```python
from build123d import *

# Parameters (mm, degrees)
CROQUIS2_R              = 1.5
SALIENTE_EXTRUIR1_DEPTH = 4
CROQUIS3_R              = 2.85
CORTAR_EXTRUIR1_DEPTH   = 1.65


with BuildPart() as part:
    # Croquis2 → Saliente-Extruir1 (new body)
    with BuildSketch(Plane.XY):
        Polygon((38.497217209, -204.70543153), (46.497217209, -204.70543153), (46.497217209, -193.70543153), (61.497217209, -193.70543153), (61.497217209, -185.70543153), (46.497217209, -185.70543153), (46.497217209, -174.70543153), (38.497217209, -174.70543153), align=None)
        with Locations((42.497217209, -189.70543153)):
            Circle(CROQUIS2_R, mode=Mode.SUBTRACT)
        with Locations((42.497217209, -199.20543153)):
            Circle(CROQUIS2_R, mode=Mode.SUBTRACT)
        with Locations((57.497217209, -189.70543153)):
            Circle(CROQUIS2_R, mode=Mode.SUBTRACT)
        with Locations((49.997217209, -189.70543153)):
            Circle(CROQUIS2_R, mode=Mode.SUBTRACT)
        with Locations((42.497217209, -180.20543153)):
            Circle(CROQUIS2_R, mode=Mode.SUBTRACT)
    extrude(amount=SALIENTE_EXTRUIR1_DEPTH)

    # Croquis3 → Cortar-Extruir1 (cut)
    with BuildSketch(Plane.XY.offset(4)):
        with Locations((42.497217209, -199.20543153)):
            Circle(CROQUIS3_R)
        with Locations((42.497217209, -189.70543153)):
            Circle(CROQUIS3_R)
        with Locations((42.497217209, -180.20543153)):
            Circle(CROQUIS3_R)
        with Locations((49.997217209, -189.70543153)):
            Circle(CROQUIS3_R)
        with Locations((57.497217209, -189.70543153)):
            Circle(CROQUIS3_R)
    extrude(amount=-CORTAR_EXTRUIR1_DEPTH, mode=Mode.SUBTRACT)


solid = part.part
```
The listing builds one solid part. Answer for the finished solid, in the listing's coordinates (mm). A direction names the side the tool comes from. Coordinates: 2 decimals unless noted, no trailing zeros. Loops run counter-clockwise (first coordinate to the right, second up) from the corner with the lowest first, then second, coordinate; pieces in that order, holes last. Notation, with made-up numbers: (-39.75, -38.75) - (-29.75, -38.75) arc R20 ccw to (-29.75, -34.75) - close; hole circle Ø3 at (-13, 46). An arc over 180 degrees is marked (long way). Write item = value, one per line.
1) Section B-B (y = -200) is taken. Determine the outline of the cut face in (x, z), plus the area to 3 significant figures.
Responses:
outline = (38.5, 0) - (41.22, 0) - (41.22, 2.35) - (39.76, 2.35) - (39.76, 4) - (38.5, 4) - close; (43.77, 0) - (46.5, 0) - (46.5, 4) - (45.23, 4) - (45.23, 2.35) - (43.77, 2.35) - close
area = 17.0 mm^2
2) Section D-D (y = -189) is taken. Determine the outline of the cut face in (x, z).
Responses:
outline = (38.5, 0) - (41.17, 0) - (41.17, 2.35) - (39.74, 2.35) - (39.74, 4) - (38.5, 4) - close; (43.82, 0) - (48.67, 0) - (48.67, 2.35) - (47.24, 2.35) - (47.24, 4) - (45.26, 4) - (45.26, 2.35) - (43.82, 2.35) - close; (51.32, 0) - (56.17, 0) - (56.17, 2.35) - (54.74, 2.35) - (54.74, 4) - (52.76, 4) - (52.76, 2.35) - (51.32, 2.35) - close; (58.82, 0) - (61.5, 0) - (61.5, 4) - (60.26, 4) - (60.26, 2.35) - (58.82, 2.35) - close
3) Each of these flat-tipped pins is pushed along its axis until it touches: P1, Ø1.2, axis at y = -201, z = 2.5, coming from the +X side; P2, Ø3.5, axis at x = 42.5, y = -189.71, coming from the +Z side; P3, Ø1.2, axis at x = 54, z = 1.5, coming from the -Y side. Where does it stop, or does it pass through?
Responses:
P1 = 46.5
P2 = 2.35
P3 = -193.71
4) Determine the mould class of faces 4 (the face through (46.497, -199, 2)), 5 (the face through (54, -185.705, 2)), 6 (the face through (43.883, -190.28, 1.159)) for opening direction X: pulls with the +X half, pulls with the -X half, needs draft (parallel to the pull), parting line crosses it, or undercut.
Responses:
face_4 = pulls with the +X half
face_5 = needs draft
face_6 = undercut
5) Section C-C (z = 3.5) is taken. Determine the outline of the cut face in (x, y), plus the area to 3 significant figures.
Responses:
outline = (38.5, -204.71) - (46.5, -204.71) - (46.5, -193.71) - (61.5, -193.71) - (61.5, -185.71) - (46.5, -185.71) - (46.5, -174.71) - (38.5, -174.71) - close; hole circle Ø5.7 at (42.5, -199.21); hole circle Ø5.7 at (42.5, -189.71); hole circle Ø5.7 at (42.5, -180.21); hole circle Ø5.7 at (50, -189.71); hole circle Ø5.7 at (57.5, -189.71)
area = 232 mm^2
6) Find the intervals of material crossed by line 1 along X through (y, z) = (-190.25, 3.7); line 2 along Y through (x, z) = (41, 3.55); line 3 along Y through (x, z) = (45, 3), in increasing order.
Responses:
line_1 = 38.5 to 39.7, 45.29 to 47.2, 52.79 to 54.7, 60.29 to 61.5
line_2 = -204.71 to -201.63, -196.78 to -192.13, -187.28 to -182.63, -177.78 to -174.71
line_3 = -204.71 to -200.57, -197.84 to -191.07, -188.34 to -181.57, -178.84 to -174.71
7) Section A-A (x = 50) is taken. Determine the outline of the cut face in (y, z), plus the area to 3 significant figures.
Responses:
outline = (-193.71, 0) - (-191.21, 0) - (-191.21, 2.35) - (-192.56, 2.35) - (-192.56, 4) - (-193.71, 4) - close; (-188.21, 0) - (-185.71, 0) - (-185.71, 4) - (-186.86, 4) - (-186.86, 2.35) - (-188.21, 2.35) - close
area = 15.5 mm^2
8) Which of the six approach directions +Z, -Z, +X, -X, +Y, -Y give full straight-line access (tool end or side, diameter ignored) to faces 1 (the face through (54, -193.705, 2)), 2 (the face through (43.812, -201.734, 3.187)), 3 (the face through (43, -174.705, 2))?
Responses:
face_1 = +Z, -Z, +X, -Y
face_2 = +Z
face_3 = +Z, -Z, +X, -X, +Y
